```python
from build123d import *

# Parameters (mm, degrees)
SKETCH1_W                        = 300
SKETCH1_H                        = 300
BOSS_EXTRUDE1_DEPTH              = 30
F_12_0MM_DOWEL_HOLE2_D           = 12
F_12_0MM_DOWEL_HOLE2_DEPTH       = 10
F_12_0MM_DOWEL_HOLE2_CSINK_D     = 12.05
F_12_0MM_DOWEL_HOLE2_CSINK_ANGLE = 90
F_12_0MM_DOWEL_HOLE2_TIP         = 3.605163714
F_12_0MM_DOWEL_HOLE3_D           = 12
F_12_0MM_DOWEL_HOLE3_DEPTH       = 10
F_12_0MM_DOWEL_HOLE3_CSINK_D     = 12.05
F_12_0MM_DOWEL_HOLE3_CSINK_ANGLE = 90
F_12_0MM_DOWEL_HOLE3_TIP         = 3.605163714
FILLET1_R                        = 30
CHAMFER1_SIZE                    = 10


with BuildPart() as part:
    # Sketch1 → Boss-Extrude1 (new body)
    with BuildSketch(Plane(origin=(0, 0, 0), x_dir=(1, 0, 0), z_dir=(0, 1, 0))):
        Rectangle(SKETCH1_W, SKETCH1_H)
    extrude(amount=BOSS_EXTRUDE1_DEPTH)

    # Ø12.0mm Dowel Hole2
    with Locations(Plane(origin=(0, 30, 0), x_dir=(1, 0, 0), z_dir=(0, 1, 0))):
        with Locations((-112.5, 112.5), (112.5, 112.5), (112.5, -112.5), (-112.5, -112.5)):
            CounterSinkHole(F_12_0MM_DOWEL_HOLE2_D / 2, F_12_0MM_DOWEL_HOLE2_CSINK_D / 2, depth=F_12_0MM_DOWEL_HOLE2_DEPTH, counter_sink_angle=F_12_0MM_DOWEL_HOLE2_CSINK_ANGLE)
            with Locations((0, 0, -(F_12_0MM_DOWEL_HOLE2_DEPTH + F_12_0MM_DOWEL_HOLE2_TIP / 2))):  # 118° drill point
                Cone(0, F_12_0MM_DOWEL_HOLE2_D / 2, F_12_0MM_DOWEL_HOLE2_TIP, mode=Mode.SUBTRACT)

    # Ø12.0mm Dowel Hole3
    with Locations(Plane(origin=(0, 0, 0), x_dir=(-1, 0, 0), z_dir=(0, -1, 0))):
        with Locations((-125, 125), (125, 125), (125, -125), (-125, -125)):
            CounterSinkHole(F_12_0MM_DOWEL_HOLE3_D / 2, F_12_0MM_DOWEL_HOLE3_CSINK_D / 2, depth=F_12_0MM_DOWEL_HOLE3_DEPTH, counter_sink_angle=F_12_0MM_DOWEL_HOLE3_CSINK_ANGLE)
            with Locations((0, 0, -(F_12_0MM_DOWEL_HOLE3_DEPTH + F_12_0MM_DOWEL_HOLE3_TIP / 2))):  # 118° drill point
                Cone(0, F_12_0MM_DOWEL_HOLE3_D / 2, F_12_0MM_DOWEL_HOLE3_TIP, mode=Mode.SUBTRACT)

    # Fillet1
    fillet1_edges = [part.edges().sort_by_distance(p)[0] for p in [
        (150, 15, 150),
        (-150, 15, 150),
        (-150, 15, -150),
        (150, 15, -150),
    ]]
    fillet(fillet1_edges, radius=FILLET1_R)

    # Chamfer1
    chamfer1_edges = [part.edges().sort_by_distance(p)[0] for p in [
        (150, 30, 0),
        (0, 30, 150),
        (0, 30, -150),
        (-150, 30, 0),
        (-141.213203436, 30, 141.213203436),
        (141.213203436, 30, -141.213203436),
        (-141.213203436, 30, -141.213203436),
        (141.213203436, 30, 141.213203436),
    ]]
    chamfer(chamfer1_edges, length=CHAMFER1_SIZE)


solid = part.part
```
Geometry check sheet. Reference: the model listing, model coordinates, mm. A direction names the side the tool comes from. Coordinates: 2 decimals unless noted, no trailing zeros. One line per item, written item: value. Start each with the question number.
(1) Tool access check on faces 1 (the face through (119, 5, -125)), 2 (the face through (116.92, 24.92, -116.56)), 3 (the face through (-141.445, 10.14, 140.979)). Record the directions out of +Z, -Z, +X, -X, +Y, -Y that give a thin tool (end or side, any length) a straight path to the whole face; none if there is none.
(2) Depth check by flat-ended pin: pin 1 (7 mm diameter, centred on x = 112.5, z = 112.5, fed in from +Y); pin 2 (9.5 mm diameter, centred on x = 125, z = -125, fed in from -Y); pin 3 (9.5 mm diameter, centred on x = -112.5, z = 112.5, fed in from +Y). Enter the tip coordinate at first touch or a pass-through.
(3) Release check for a two-part mould opening along X. For faces 4 (the face through (-2, 0, -2)), 5 (the face through (-129.76, 5.08, -121.35)), 6 (the face through (140.979, 10.14, -141.445)) record: released by +X, released by -X, zero draft, split by the parting line, or undercut.
(4) Scan lines: line 1 along Z through (x, y) = (125, 7.5); line 2 along Z through (x, y) = (-112.5, 23.5); line 3 along X through (y, z) = (23, 112.5). Record each from-to range of solid material in increasing order. Write a range as [from, to].
Filled sheet:
1. face 1: -Y
1. face 2: +Y
1. face 3: +Z, -X, +Y, -Y
2. pin 1: y = 18.5
2. pin 2: y = 10.75
2. pin 3: y = 19.25
3. face 4: zero draft
3. face 5: undercut
3. face 6: released by +X
4. line 1: [-149.58, -131], [-119, 119], [131, 149.58]
4. line 2: [-146.5, -118.5], [-106.5, 106.5], [118.5, 146.5]
4. line 3: [-147, -118.5], [-106.5, 106.5], [118.5, 147]
